Could you check a few things on this model? Use its own coordinates, in mm. Give positions to 0.01 mm unless a question says otherwise; leave off trailing zeros. Loops run counter-clockwise (first coordinate to the right, second up) from the corner with the lowest first, then second, coordinate; pieces in that order, holes last. Notation, with made-up numbers: M -20.75,39.5 L 29.25,39.5 A30 cw 29.25,68.5 Z; hole C -32,82 d7. An arc over 180 degrees is marked long. Answer in a Markdown table with one row per item. Add a question column.
```python
from build123d import *

# Parameters (mm, degrees)
SKETCH1_R               = 5
DOME1_FACE_RADIUS       = 5
DOME1_HEIGHT            = 5
DOME2_FACE_RADIUS       = 5
DOME2_HEIGHT            = 5
CUT_EXTRUDE2_DEPTH      = 5.404285297
CUT_EXTRUDE2_DEPTH_BACK = 289.404285297
SKETCH6_R               = 2
CUT_EXTRUDE3_DEPTH      = 68.142339226
CUT_EXTRUDE3_DEPTH_BACK = 6.72259346
CUT_EXTRUDE5_DEPTH      = 5.047319689
CUT_EXTRUDE5_DEPTH_BACK = 410.929194171
SKETCH8_R               = 2
CUT_EXTRUDE6_DEPTH      = 6.613212564
CUT_EXTRUDE6_DEPTH_BACK = 25.970742243


with BuildPart() as part:
    # Sweep1: sweep along a path in Sketch3
    with BuildLine(Plane(origin=(0, 0, 0), x_dir=(0, 0, -1), z_dir=(1, 0, 0))) as sweep1_path:
        Line((0, 0), (487.405602585, 0))
    # Sketch1 → Sweep1 (sweep)
    with BuildSketch(Plane.XY):
        Circle(SKETCH1_R)
    sweep(path=sweep1_path.line)

    # Dome1: a dome of height H over a round flat face of radius A is a cap of a sphere of radius (A * A + H * H) / (2 * H)
    dome1_r = (DOME1_FACE_RADIUS * DOME1_FACE_RADIUS + DOME1_HEIGHT * DOME1_HEIGHT) / (2 * DOME1_HEIGHT)
    dome1_base = Plane((0, 0, 0), z_dir=(0, 0, 1))
    with Locations(dome1_base.offset(DOME1_HEIGHT - dome1_r)):
        dome1_ball = Sphere(dome1_r, mode=Mode.PRIVATE)
    add(split(dome1_ball, bisect_by=dome1_base, keep=Keep.TOP, mode=Mode.PRIVATE))

    # Dome2: a dome of height H over a round flat face of radius A is a cap of a sphere of radius (A * A + H * H) / (2 * H)
    dome2_r = (DOME2_FACE_RADIUS * DOME2_FACE_RADIUS + DOME2_HEIGHT * DOME2_HEIGHT) / (2 * DOME2_HEIGHT)
    dome2_base = Plane((0, 0, -487.405602585), z_dir=(0, 0, -1))
    with Locations(dome2_base.offset(DOME2_HEIGHT - dome2_r)):
        dome2_ball = Sphere(dome2_r, mode=Mode.PRIVATE)
    add(split(dome2_ball, bisect_by=dome2_base, keep=Keep.TOP, mode=Mode.PRIVATE))

    # Sketch5 → Cut-Extrude2 (cut, two sides)
    with BuildSketch(Plane(origin=(-26.571757691, 229.275990101, -160.273085877), x_dir=(0.995516802, 0.078714536, -0.052443479), z_dir=(-0.094561415, 0.81592879, -0.570366854))) as cut_extrude2_sk:
        Polygon((22.843463066, 396.275337774), (22.1233695, 404.242954928), (25.111191904, 404.512986939), (25.831285469, 396.545369785), align=None)
    extrude(amount=CUT_EXTRUDE2_DEPTH, mode=Mode.SUBTRACT)
    extrude(cut_extrude2_sk.sketch, amount=-CUT_EXTRUDE2_DEPTH_BACK, mode=Mode.SUBTRACT)

    # Sketch6 → Cut-Extrude3 (cut, two sides)
    with BuildSketch(Plane(origin=(60.907834636, 1.64848777, -7.739724677), x_dir=(0.126296417, -0.009108801, 0.991950727), z_dir=(-0.991665366, -0.026839704, 0.126013623))) as cut_extrude3_sk:
        with Locations((-483.482341842, -6.054864831)):
            Circle(SKETCH6_R)
    extrude(amount=CUT_EXTRUDE3_DEPTH, mode=Mode.SUBTRACT)
    extrude(cut_extrude3_sk.sketch, amount=-CUT_EXTRUDE3_DEPTH_BACK, mode=Mode.SUBTRACT)

    # Sketch7 → Cut-Extrude5 (cut, two sides)
    with BuildSketch(Plane(origin=(-0.052668832, 1.714434817, 2.461288129), x_dir=(0.999845409, 0.010828351, 0.013852985), z_dir=(-0.017556277, 0.571478272, 0.820429376))) as cut_extrude5_sk:
        Polygon((-2.594541679, -4.452930477), (0.392284328, -4.172091725), (-0.280838752, 2.986826007), (-3.267664759, 2.705987255), align=None)
    extrude(amount=CUT_EXTRUDE5_DEPTH, mode=Mode.SUBTRACT)
    extrude(cut_extrude5_sk.sketch, amount=-CUT_EXTRUDE5_DEPTH_BACK, mode=Mode.SUBTRACT)

    # Sketch8 → Cut-Extrude6 (cut, two sides)
    with BuildSketch(Plane(origin=(0, 0, 0), x_dir=(0.039771244, 0.001105127, 0.9992082), z_dir=(-0.995364213, -0.087594482, 0.039715122))) as cut_extrude6_sk:
        Circle(SKETCH8_R)
    extrude(amount=CUT_EXTRUDE6_DEPTH, mode=Mode.SUBTRACT)
    extrude(cut_extrude6_sk.sketch, amount=-CUT_EXTRUDE6_DEPTH_BACK, mode=Mode.SUBTRACT)


solid = part.part
```
Item 1: Suppose I cut it at A-A (z = -194). List the corners of the cut face in (x, y) for me.
Item 2: If we mould it in two halves opening along Z, with no side actions, what happens to faces 1 (the face through (-1.08, 4.88, -247.11)), 2 (the face through (-1.679, -0.194, -5.26))? For each: +Z half, -Z half, draft (parallel to the pull), parting line (faces both ways), or undercut.
Item 3: For P1, Ø4, axis at x = 3, z = -367, coming from the +Y side; P2, Ø2, axis at x = -1.5, z = -432, coming from the -Y side; P3, Ø3, axis at x = 3.5, y = -3.5, coming from the +Z side, each with a flat end and sliding along its axis, tell me the tip position at first contact or that it passes through.
Item 4: I need wall thicknesses on L1, parallel to Z at x = -4, y = -0.5; L2, parallel to Y at x = -1, z = -235.5; L3, parallel to X at y = -0.25, z = -147. Which ranges of each line are inside material? Lowest first, please.
Values found:
| question | item | result |
|---|---|---|
| 1 | outline | C 0,0 d10 |
| 2 | face 1 | draft |
| 2 | face 2 | undercut |
| 3 | P1 | y = 4.9 |
| 3 | P2 | y = -4.97 |
| 3 | P3 | z = 3.62 |
| 4 | L1 | -490.36 to -488.87, -484.92 to -1.84, 2.16 to 2.96 |
| 4 | L2 | -4.9 to 4.9 |
| 4 | L3 | -4.99 to 4.99 |
